from build123d import *

# Parameters (mm, degrees)
F1_DEPTH      = 33.782
F1_DEPTH_BACK = 30.988
F2_W          = 23.3154920861
F2_H          = 10.7609964907
F3_DEPTH      = 133.35
F4_W          = 40.752293542
F4_H          = 22.821725624
F5_DEPTH      = 113.792
F6_R          = 6.3550530627
F6_R_2        = 5.6399455055
F6_R_3        = 6.2542744147
F6_R_4        = 6.3550538293
F7_DEPTH      = 204.978
F8_W          = 66.5587559342
F8_H          = 11.7573849857
F9_DEPTH      = 176.53


with BuildPart() as f1:
    # F0 (on Front) → F1 (new body, two sides)
    with BuildSketch(Plane.XZ) as f1_sk:
        Polygon((66.5587559342, -49.5205111802), (11.9566628709, 49.5205111802), (-66.5587559342, 49.5205111802), (-66.5587559342, -49.5205111802), align=None)
    extrude(amount=F1_DEPTH)
    extrude(f1_sk.sketch, amount=-F1_DEPTH_BACK)

    # F2 (on face) → F3 (cut)
    with BuildSketch(Plane(origin=(-66.5587559342, 0, 0), x_dir=(0, -1, 0), z_dir=(-1, 0, 0))):
        with Locations((0.0996389426, 44.1400129348)):
            Rectangle(F2_W, F2_H)
    extrude(amount=-F3_DEPTH, mode=Mode.SUBTRACT)

    # F4 (on face) → F5 (cut)
    with BuildSketch(Plane(origin=(0, 0, -49.5205111802), x_dir=(1, 0, 0), z_dir=(0, 0, -1))):
        with Locations((46.1826091632, 22.371137188)):
            Rectangle(F4_W, F4_H)
    extrude(amount=-F5_DEPTH, mode=Mode.SUBTRACT)

    # F6 (on face) → F7 (cut)
    with BuildSketch(Plane(origin=(-66.5587559342, 0, 0), x_dir=(0, -1, 0), z_dir=(-1, 0, 0))):
        with Locations((-21.3227141649, 15.6433004886)):
            Circle(F6_R)
        with Locations((-3.7862760946, 18.8317429274)):
            Circle(F6_R_2)
        with Locations((-19.927771762, -14.4476341084)):
            Circle(F6_R_3)
        with Locations((-2.5906104129, -19.6288544685)):
            Circle(F6_R_4)
    extrude(amount=-F7_DEPTH, mode=Mode.SUBTRACT)

    # F8 (on face) → F9 (cut)
    with BuildSketch(Plane.XZ.offset(33.782)):
        with Locations((-33.2793779671, -43.6418186873)):
            Rectangle(F8_W, F8_H)
    extrude(amount=-F9_DEPTH, mode=Mode.SUBTRACT)


solid = f1.part
Verification items for the finished model (mm, model axes). A direction names the side the tool comes from. Give positions to 0.01 mm unless a question says otherwise; leave off trailing zeros. Order: outer loops, then holes, each group sorted by start corner. A loop starts at its lowest first (then second) coordinate and runs counter-clockwise, first axis right, second up. Notation, with made-up numbers: M 76,-29 L 113,-29 A22 cw 113,3 Z; hole C 73.25,-17 d5. An arc over 180 degrees is marked long. Answer as a JSON object with one key per item and string values. Group by question number.
1) Scan lines: line 1 along Y through (x, z) = (-7, -18.5); line 2 along Z through (x, y) = (21.5, 2.5); line 3 along Z through (x, y) = (2.5, 16). Record each from-to range of solid material in increasing order. Write a range as [from, to].
2) Access from +Z, -Z, +X, -X, +Y, -Y to the whole of each face (thin tool, end or side, straight path). Record for faces 1 (the face through (0, -2, -44)), 2 (the face through (-25, 0, 38.76)), 3 (the face through (25.806, -22, -13)).
3) Cross-section at B-B (z = -17.5). Enter the section's corners in (x, y), then the cut area to 3 significant figures.
4) Cross-section at A-A (y = -20). Enter the section's corners in (x, z), then the cut area to 3 significant figures.
5) Depth check by flat-ended pin: pin 1 Ø7.5 at (y, z) = (2.59, -19.63) entering from -X; pin 2 Ø1.5 at (x, y) = (-27, 11.5) entering from +Z; pin 3 Ø7 at (x, y) = (-34.5, 0.5) entering from +Z; pin 4 Ø2 at (x, y) = (-37, -1.5) entering from -Z. Enter the tip coordinate at first touch or a pass-through.
6) Cross-section at C-C (x = -26). Enter the section's corners in (y, z), then the cut area to 3 significant figures.
7) Mould release check, pull along Z, two halves, no side actions. Record for faces 4 (the face through (33, 5, -49.521)), 5 (the face through (-8.765, 20.742, -8.247)), 6 (the face through (-16, 30.988, 1)): released by +Z, released by -Z, zero draft, split by the parting line, or undercut.
8) Cross-section at D-D (y = 6). Enter the section's corners in (x, z), then the cut area to 3 significant figures.
Result sheet:
{
 "1": {"line 1": "y = [-33.78, -3.66], [8.84, 15.16], [24.69, 30.99]", "line 2": "z = [-49.52, -25.98], [-13.27, 13.34], [24.32, 32.21]", "line 3": "z = [-49.52, -19.31], [-9.58, 12.17], [19.12, 49.52]"},
 "2": {"face 1": "-Z, -X, +Y, -Y", "face 2": "+Z, +X, -X", "face 3": "+Z, -Z, +X, -Y"},
 "3": {"outline": "M -66.56,-33.78 L 25.81,-33.78 L 25.81,-10.96 L 48.91,-10.96 L 48.91,-3.4 L -66.56,-3.4 Z; M -66.56,8.58 L 48.91,8.58 L 48.91,14.47 L -66.56,14.47 Z; M -66.56,25.39 L 48.91,25.39 L 48.91,30.99 L -66.56,30.99 Z", "area": "4,310 mm2"},
 "4": {"outline": "M -66.56,-37.76 L 0,-37.76 L 0,-49.52 L 25.81,-49.52 L 25.81,24.4 L 11.96,49.52 L -66.56,49.52 Z", "area": "8,190 mm2"},
 "5": {"pin 1": "passes through", "pin 2": "stops at z = 49.52", "pin 3": "stops at z = 38.76", "pin 4": "stops at z = -37.76"},
 "6": {"outline": "M -33.78,-37.76 L 30.99,-37.76 L 30.99,49.52 L 11.56,49.52 L 11.56,38.76 L -11.76,38.76 L -11.76,49.52 L -33.78,49.52 Z; hole C 2.59,-19.63 d12.71; hole C 3.79,18.83 d11.28; hole C 19.93,-14.45 d12.51; hole C 21.32,15.64 d12.71", "area": "4,930 mm2"},
 "7": {"face 4": "released by -Z", "face 5": "undercut", "face 6": "zero draft"},
 "8": {"outline": "M -66.56,-37.76 L 0,-37.76 L 0,-49.52 L 66.56,-49.52 L 53.04,-24.99 L -66.56,-24.99 Z; M -66.56,-14.27 L 47.12,-14.27 L 31.74,13.64 L -66.56,13.64 Z; M -66.56,24.02 L 26.02,24.02 L 17.89,38.76 L -66.56,38.76 Z", "area": "6,580 mm2"}
}
